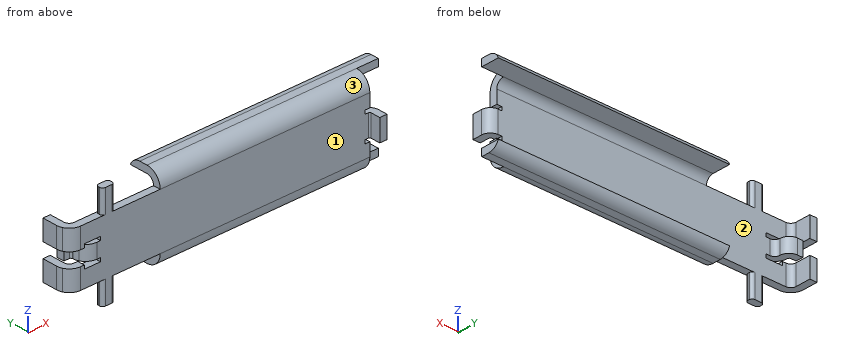
```python
from build123d import *

# Parameters (mm, degrees)
BASE_FLANGE2_DEPTH              = 45
FRONT_CUT_DEPTH                 = 2
FRONT_STRIP_W                   = 4.4
FRONT_STRIP_H                   = 1
FRONT_STRIP_CUT_DEPTH           = 3
FRONT_RELIEF_W                  = 4.9
FRONT_RELIEF_H                  = 0.5
FRONT_RELIEF_CUT_DEPTH          = 1
FRONT_DEPTH                     = 3
BACK_CUT_DEPTH                  = 13
GUIDING_PINS_DEPTH              = 7
FILLET3_R                       = 1.5
BACK_START                      = -3.8
BACK_2_BENDS_DEPTH              = 7.6
BACK_2_BENDS_2_DEPTH            = 7.6
MIDDLE_CUT_DEPTH                = 46.675485766
MIDDLE_CUT_DEPTH_BACK           = 46.675485766
SKETCH32_W                      = 2.5
SKETCH32_H                      = 2
MIDDLE_START                    = -1.5
MIDDLE_SPRING_1_DEPTH           = 3
MIDDLE_SPRING_1_2_DEPTH         = 0.5
MIDDLE_START_2                  = 1
MIDDLE_SPRING_1_3_DEPTH         = 0.5
MIDDLE_START_3                  = -1
MIDDLE_SPRING_1_4_DEPTH         = 2
MIDDLE_SPRING_2_STRIP_W         = 4.5
MIDDLE_SPRING_2_STRIP_H         = 1
MIDDLE_SPRING_2_STRIP_CUT_DEPTH = 2
MIDDLE_SPRING_2_DEPTH           = 2
SKETCH50_W                      = 1
SKETCH50_H                      = 2.8
BACK_2_BENDS_EXTENSION_DEPTH    = 2


# Read off the part's stored shape, not the designer's step: back cut, back 2 bends, middle spring 1
# Sheet-metal steps are written as plain solids
with BuildPart() as part:
    # Sketch6 → Base-Flange2 (new body)
    with BuildSketch(Plane(origin=(0, 0, 0), x_dir=(0, 0, -1), z_dir=(1, 0, 0))):
        with BuildLine():
            Line((-4.8, 3.5), (-4.8, 1))
            ThreePointArc((-4.8, 1), (-4.507106781, 0.292893219), (-3.8, 0))
            Line((-3.8, 0), (3.8, 0))
            ThreePointArc((3.8, 0), (4.507106781, 0.292893219), (4.8, 1))
            Line((4.8, 1), (4.8, 3.5))
            Line((4.8, 3.5), (5.8, 3.5))
            Line((5.8, 3.5), (5.8, 1))
            ThreePointArc((5.8, 1), (5.214213562, -0.414213562), (3.8, -1))
            Line((3.8, -1), (-3.8, -1))
            ThreePointArc((-3.8, -1), (-5.214213562, -0.414213562), (-5.8, 1))
            Line((-5.8, 1), (-5.8, 3.5))
            Line((-5.8, 3.5), (-4.8, 3.5))
        make_face()
    extrude(amount=BASE_FLANGE2_DEPTH)

    # Sketch51 → front cut (cut)
    with BuildSketch(Plane.XZ.offset(1)):
        Polygon((42, 1.5), (43, 1.5), (43, -1.5), (42, -1.5), (42, -6), (46, -6), (46, -1.5), (45, -1.5), (45, 1.5), (46, 1.5), (46, 6), (42, 6), align=None)
    extrude(amount=-FRONT_CUT_DEPTH, mode=Mode.SUBTRACT)

    # front strip (across the edge) → front strip cut (cut)
    with BuildSketch(Plane(origin=(43, -1, -1.5), x_dir=(-1, 0, 0), z_dir=(0, 0, 1))):
        with Locations((-1, -0.5)):
            Rectangle(FRONT_STRIP_W, FRONT_STRIP_H)
    extrude(amount=FRONT_STRIP_CUT_DEPTH, mode=Mode.SUBTRACT)

    # front relief (on the sheet) → front relief cut (cut)
    with BuildSketch(Plane(origin=(41.8, -1, -1.5), x_dir=(-1, 0, 0), z_dir=(0, -1, 0))):
        with Locations((-1.95, 0.25)):
            Rectangle(FRONT_RELIEF_W, FRONT_RELIEF_H)
        with Locations((-1.95, -3.25)):
            Rectangle(FRONT_RELIEF_W, FRONT_RELIEF_H)
    extrude(amount=-FRONT_RELIEF_CUT_DEPTH, mode=Mode.SUBTRACT)

    # front section (across the edge) → front (add)
    with BuildSketch(Plane(origin=(43, -1, -1.5), x_dir=(-1, 0, 0), z_dir=(0, 0, 1))):
        with BuildLine():
            Line((0, 0.2), (0, 1.5))
            Line((0, 1.5), (1, 1.5))
            Line((1, 1.5), (1, 0.2))
            ThreePointArc((1, 0.2), (1.058578644, 0.058578644), (1.2, 0))
            Line((1.2, 0), (1.2, -1))
            ThreePointArc((1.2, -1), (0.351471863, -0.648528137), (0, 0.2))
        make_face()
    extrude(amount=FRONT_DEPTH)

    # back cut outline → back cut (cut)
    with BuildSketch(Plane.YZ):
        with BuildLine():
            Line((-1, 3.8), (0, 3.8))
            ThreePointArc((0, 3.8), (0.292893219, 4.507106781), (1, 4.8))
            Line((1, 4.8), (3.5, 4.8))
            Line((3.5, 4.8), (3.5, 5.8))
            Line((3.5, 5.8), (1, 5.8))
            ThreePointArc((1, 5.8), (-0.414213562, 5.214213562), (-1, 3.8))
        make_face()
        with BuildLine():
            ThreePointArc((1, -4.8), (0.292893219, -4.507106781), (0, -3.8))
            Line((0, -3.8), (-1, -3.8))
            ThreePointArc((-1, -3.8), (-0.414213562, -5.214213562), (1, -5.8))
            Line((1, -5.8), (3.5, -5.8))
            Line((3.5, -5.8), (3.5, -4.8))
            Line((3.5, -4.8), (1, -4.8))
        make_face()
    extrude(amount=BACK_CUT_DEPTH, mode=Mode.SUBTRACT)

    # Sketch27 → guiding pins (add, symmetric)
    with BuildSketch(Plane.XY):
        with BuildLine():
            Line((5.4, 0), (6.3, 0))
            ThreePointArc((6.3, 0), (6.582842712, -0.117157288), (6.7, -0.4))
            Line((6.7, -0.4), (6.7, -0.6))
            ThreePointArc((6.7, -0.6), (6.582842712, -0.882842712), (6.3, -1))
            Line((6.3, -1), (5.4, -1))
            ThreePointArc((5.4, -1), (5.117157288, -0.882842712), (5, -0.6))
            Line((5, -0.6), (5, -0.4))
            ThreePointArc((5, -0.4), (5.117157288, -0.117157288), (5.4, 0))
        make_face()
    extrude(amount=GUIDING_PINS_DEPTH, both=True)

    # Fillet3
    # the kernel refuses this fillet: 1.5 mm, written as the material it takes off along each edge
    with BuildSketch(Plane(origin=(9.464466094, 3.5, 5.8), x_dir=(0, -1, 0), z_dir=(1, 0, 0))) as fillet3_piece_1:
        with BuildLine():
            CenterArc((1.414213562, 1.5), FILLET3_R, 199.471220634, 70.528779366)
            Line((0, 1), (-0.028284271, 0.99))
            ThreePointArc((-0.028284271, 0.99), (-0.03, 0.5), (-0.03, 0))
            Line((-0.03, 0), (0, -0.03))
            Line((0, -0.03), (1.414213562, -0.03))
            Line((1.414213562, -0.03), (1.414213562, 0))
        make_face()
    extrude(amount=39.071067812, mode=Mode.SUBTRACT)
    with BuildSketch(Plane(origin=(9.464466094, 3.5, -5.8), x_dir=(0, -1, 0), z_dir=(1, 0, 0))) as fillet3_piece_2:
        with BuildLine():
            CenterArc((1.414213562, -1.5), FILLET3_R, 90, 70.528779366)
            Line((0, -1), (-0.028284271, -0.99))
            ThreePointArc((-0.028284271, -0.99), (-0.03, -0.5), (-0.03, 0))
            Line((-0.03, 0), (0, 0.03))
            Line((0, 0.03), (1.414213562, 0.03))
            Line((1.414213562, 0.03), (1.414213562, 0))
        make_face()
    extrude(amount=39.071067812, mode=Mode.SUBTRACT)

    # back 2 bends outline → back 2 bends (cut)
    with BuildSketch(Plane.XY.offset(BACK_START)):
        with BuildLine():
            Line((0, -1), (2, -1))
            ThreePointArc((2, -1), (1.068173836, -0.728828115), (0.42735891, 0))
            Line((0.42735891, 0), (0, 0))
            Line((0, 0), (0, -1))
        make_face()
    extrude(amount=BACK_2_BENDS_DEPTH, mode=Mode.SUBTRACT)

    # back 2 bends 2 outline → back 2 bends 2 (add)
    with BuildSketch(Plane.XY.offset(BACK_START)):
        with BuildLine():
            ThreePointArc((0.2634, 0.7366), (0.304885243, 0.359286442), (0.42735891, 0))
            Line((0.42735891, 0), (2, 0))
            ThreePointArc((2, 0), (1.479145145, 0.215745145), (1.2634, 0.7366))
            Line((1.2634, 0.7366), (1.2634, 0.794153262))
            Line((1.2634, 0.794153262), (0.2634, 0.794153262))
            Line((0.2634, 0.794153262), (0.2634, 0.7366))
        make_face()
    extrude(amount=BACK_2_BENDS_2_DEPTH)

    # Sketch32 → middle cut (cut, two sides: drawn at the far end of the back side and taken through both)
    with BuildSketch(Plane(origin=(0, 0, 0), x_dir=(1, 0, 0), z_dir=(0, 1, 0)).offset(-MIDDLE_CUT_DEPTH_BACK)):
        with Locations((1.25, 0)):
            Rectangle(SKETCH32_W, SKETCH32_H)
    extrude(amount=MIDDLE_CUT_DEPTH + MIDDLE_CUT_DEPTH_BACK, mode=Mode.SUBTRACT)

    # middle spring 1 outline → middle spring 1 (cut)
    with BuildSketch(Plane.XY.offset(MIDDLE_START)):
        with BuildLine():
            Line((2.5, 0), (2.5, -1))
            Line((2.5, -1), (4.2366, -1))
            ThreePointArc((4.2366, -1), (3.304773836, -0.728828115), (2.66395891, 0))
            Line((2.66395891, 0), (2.5, 0))
        make_face()
    extrude(amount=MIDDLE_SPRING_1_DEPTH, mode=Mode.SUBTRACT)

    # middle spring 1 2 outline → middle spring 1 2 (cut)
    with BuildSketch(Plane.XY.offset(MIDDLE_START)):
        with BuildLine():
            ThreePointArc((2.66395891, 0), (3.304773836, -0.728828115), (4.2366, -1))
            Line((4.2366, -1), (4.7366, -1))
            Line((4.7366, -1), (4.7366, 0))
            Line((4.7366, 0), (2.66395891, 0))
        make_face()
    extrude(amount=MIDDLE_SPRING_1_2_DEPTH, mode=Mode.SUBTRACT)

    # middle spring 1 3 outline → middle spring 1 3 (cut)
    with BuildSketch(Plane.XY.offset(MIDDLE_START_2)):
        with BuildLine():
            ThreePointArc((2.66395891, 0), (3.304773836, -0.728828115), (4.2366, -1))
            Line((4.2366, -1), (4.7366, -1))
            Line((4.7366, -1), (4.7366, 0))
            Line((4.7366, 0), (2.66395891, 0))
        make_face()
    extrude(amount=MIDDLE_SPRING_1_3_DEPTH, mode=Mode.SUBTRACT)

    # middle spring 1 4 outline → middle spring 1 4 (add)
    with BuildSketch(Plane.XY.offset(MIDDLE_START_3)):
        with BuildLine():
            ThreePointArc((2.5, 0.7366), (2.541485243, 0.359286442), (2.66395891, 0))
            Line((2.66395891, 0), (4.2366, 0))
            ThreePointArc((4.2366, 0), (3.715745145, 0.215745145), (3.5, 0.7366))
            Line((3.5, 0.7366), (3.5, 2))
            Line((3.5, 2), (2.5, 2))
            Line((2.5, 2), (2.5, 0.7366))
        make_face()
    extrude(amount=MIDDLE_SPRING_1_4_DEPTH)

    # middle spring 2 strip (across the edge) → middle spring 2 strip cut (cut)
    with BuildSketch(Plane(origin=(2.5, 2, 1), x_dir=(0, -1, 0), z_dir=(0, 0, -1))):
        with Locations((-1, -0.5)):
            Rectangle(MIDDLE_SPRING_2_STRIP_W, MIDDLE_SPRING_2_STRIP_H)
    extrude(amount=MIDDLE_SPRING_2_STRIP_CUT_DEPTH, mode=Mode.SUBTRACT)

    # middle spring 2 section (across the edge) → middle spring 2 (add)
    with BuildSketch(Plane(origin=(2.5, 2, 1), x_dir=(0, -1, 0), z_dir=(0, 0, -1))):
        with BuildLine():
            Line((0, 0.25), (0, 1))
            Line((0, 1), (1, 1))
            Line((1, 1), (1, 0.25))
            ThreePointArc((1, 0.25), (1.073223305, 0.073223305), (1.25, 0))
            Line((1.25, 0), (1.25, -1))
            ThreePointArc((1.25, -1), (0.366116524, -0.633883476), (0, 0.25))
        make_face()
    extrude(amount=MIDDLE_SPRING_2_DEPTH)

    # Sketch50 → back 2 bends extension (add)
    with BuildSketch(Plane(origin=(0, 0.794153262, 0), x_dir=(1, 0, 0), z_dir=(0, 1, 0))):
        with Locations((0.7634, -2.4)):
            Rectangle(SKETCH50_W, SKETCH50_H)
        with Locations((0.7634, 2.4)):
            Rectangle(SKETCH50_W, SKETCH50_H)
    extrude(amount=BACK_2_BENDS_EXTENSION_DEPTH)


solid = part.part
```
Part model, mm, in its own coordinate system. Face numbers are marked on the shaded views. Give positions to 0.01 mm unless a question says otherwise; leave off trailing zeros. Loops run counter-clockwise (first coordinate to the right, second up) from the corner with the lowest first, then second, coordinate; pieces in that order, holes last. Notation, with made-up numbers: M -10,43 L 44,43 A19 cw 44,58 Z; hole C -7.5,4 d6. An arc over 180 degrees is marked long. Return JSON: item names as keys, results as strings.
1) Saw through at C-C, the plane x = 22. List the corners of the cut face in (y, z), then the cut area to 3 significant figures.
Calculated:
{"outline": "M -1,-3.8 A2 ccw 1,-5.8 L 2.09,-5.8 A1.5 ccw 3.5,-4.8 L 1,-4.8 A1 cw 0,-3.8 L 0,3.8 A1 cw 1,4.8 L 3.5,4.8 A1.5 ccw 2.09,5.8 L 1,5.8 A2 ccw -1,3.8 Z", "area": "16.5 mm2"}
2) Saw through at A-A, the plane y = 1.5. List the corners of the cut face in (x, z).
Calculated:
{"outline": "M 0.26,-3.8 L 1.26,-3.8 L 1.26,-1 L 0.26,-1 Z; M 0.26,1 L 1.26,1 L 1.26,3.8 L 0.26,3.8 Z; M 1.5,-1 L 3.25,-1 L 3.25,1 L 1.5,1 Z; M 13,-5.8 L 45,-5.8 L 45,-4.8 L 13,-4.8 Z; M 13,4.8 L 45,4.8 L 45,5.8 L 13,5.8 Z"}
3) Drill centre lines: line 1 (Z direction, x = 37.5, y = 1.25); line 2 (X direction, y = 0.75, z = -5.5); line 3 (X direction, y = 1.25, z = 1.75). Where is each one in solid material? Low to high.
Calculated:
{"line 1": "z = -5.8 to -4.8, 4.8 to 5.8", "line 2": "x = 13 to 42", "line 3": "x = 0.26 to 1.26"}
4) Flat gauge pins, fed straight in: pin 1 Ø0.6 at (x, y) = (41.5, -0.5) entering from -Z; pin 2 Ø3 at (x, z) = (25.5, -1.5) entering from +Y; pin 3 Ø0.8 at (x, z) = (43.5, -5.5) entering from -Y. Where does each tip first touch, or does it go through?
Calculated:
{"pin 1": "stops at z = -5.4", "pin 2": "stops at y = 0", "pin 3": "stops at y = 1"}
5) Saw through at D-D, the plane z = 3.25. List the corners of the cut face in (x, y).
Calculated:
{"outline": "M 0.26,0.74 A1.74 ccw 2,-1 L 42,-1 L 42,0 L 2,0 A0.74 cw 1.26,0.74 L 1.26,2.79 L 0.26,2.79 Z"}
6) Pull direction Z, two halves, no side cores. Call the marked faces 1, 2 and 3: released by +Z, released by -Z, zero draft, split by the parting line, or undercut.
Calculated:
{"face 1": "zero draft", "face 2": "undercut", "face 3": "released by +Z"}
